Drawing for the job (mm, zero at the part's lowest x, y, z). A direction names the side the tool comes from. Coordinates: 2 decimals unless noted, no trailing zeros. Write each loop counter-clockwise with the first axis right and the second up, starting at its lowest first coordinate (ties: lowest second). Pieces come first, ordered by that corner, then holes. Notation, with made-up numbers: M 46,64.25 L 97,64.25 A16 ccw 97,77.25 Z; hole C 74.25,-38 d1. An arc over 180 degrees is marked long. Put each result on its own line as item: value. Start each with the question number.
Q1. Drop flat-ended pins along their axis: pin 1 (8 mm diameter, centred on x = 34, y = 34, fed in from -Z); pin 2 (8 mm diameter, centred on x = 19, y = 75, fed in from +Z); pin 3 (4 mm diameter, centred on x = 7, z = 36, fed in from +Y). Give the stop position or say it passes through.
Q2. Cut at C-C (y = 94.5). Write the cut outline in (x, z).
Q3. Cut at A-A (x = 20). Write the cut outline in (y, z), then the cut area to 3 significant figures.
Q4. Which spindle directions (+Z, -Z, +X, -X, +Y, -Y) get a long thin tool onto all of the face, cutting with end or side? Do the marked faces 1, 2 and 3. Say none if no direction does.
Q5. Cut at D-D (z = 33). Write the cut outline in (x, y).
Q6. Drill centre lines: line 1 along Y through (x, z) = (4, 12.5); line 2 along Y through (x, z) = (37.5, 27.5); line 3 along Z through (x, y) = (11, 57). Where is each one in solid material? Low to high.
Q7. Cut at B-B (z = 20). Write the cut outline in (x, y), then the cut area to 3 significant figures.
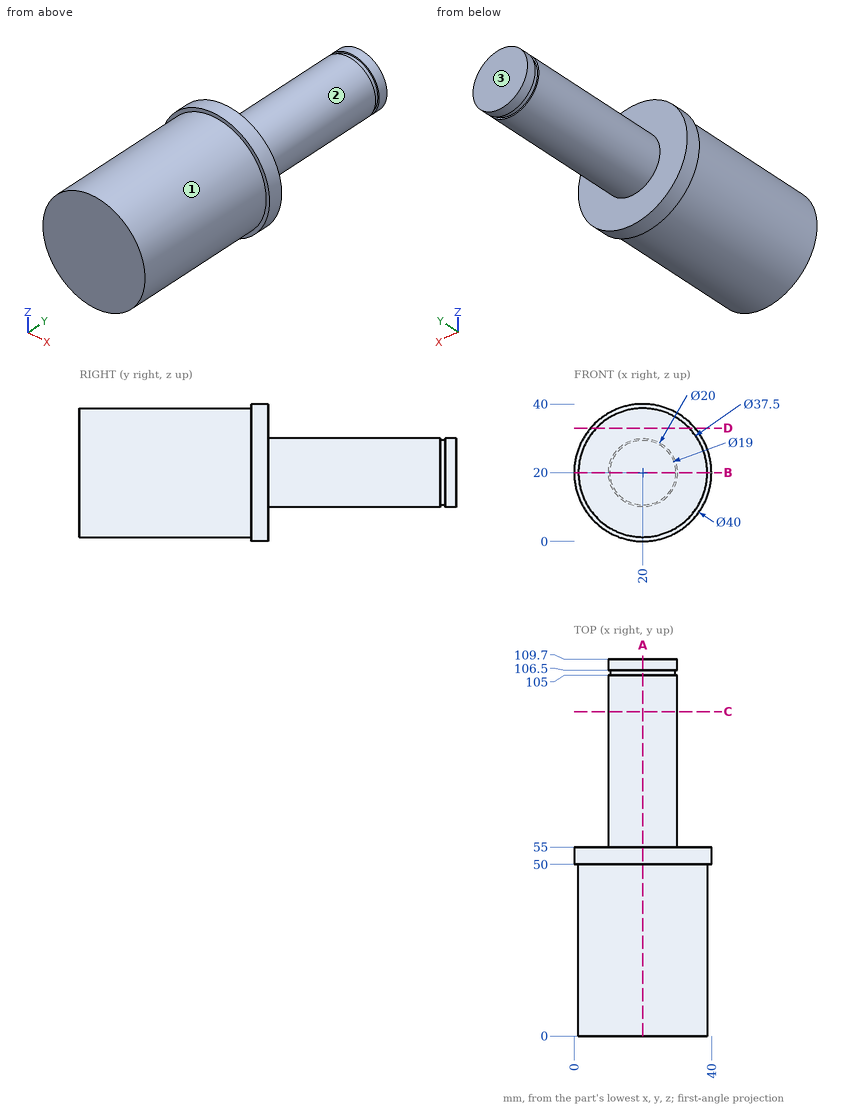
Computed values:
1. pin 1: z = 4.14
1. pin 2: z = 30
1. pin 3: y = 55
2. outline: C 20,20 d20
3. outline: M 0,1.25 L 50,1.25 L 50,0 L 55,0 L 55,10 L 105,10 L 105,10.5 L 106.5,10.5 L 106.5,10 L 109.7,10 L 109.7,30 L 106.5,30 L 106.5,29.5 L 105,29.5 L 105,30 L 55,30 L 55,40 L 50,40 L 50,38.75 L 0,38.75 Z
3. area: 3,170 mm2
4. face 1: -Y
4. face 2: +Y
4. face 3: +Z, -Z, +X, -X, +Y
5. outline: M 4.8,50 L 6.49,50 L 6.49,0 L 33.51,0 L 33.51,50 L 35.2,50 L 35.2,55 L 4.8,55 Z
6. line 1: 0 to 55
6. line 2: 50 to 55
6. line 3: 15.64 to 24.36
7. outline: M 0,50 L 1.25,50 L 1.25,0 L 38.75,0 L 38.75,50 L 40,50 L 40,55 L 30,55 L 30,105 L 29.5,105 L 29.5,106.5 L 30,106.5 L 30,109.7 L 10,109.7 L 10,106.5 L 10.5,106.5 L 10.5,105 L 10,105 L 10,55 L 0,55 Z
7. area: 3,170 mm2
